Source: CAD feature listing. Evaluate the final solid. Frame: model axes, mm. Face numbers are marked on the shaded views. A direction names the side the tool comes from. Give positions to 0.01 mm unless a question says otherwise; leave off trailing zeros. Order: outer loops, then holes, each group sorted by start corner. A loop starts at its lowest first (then second) coordinate and runs counter-clockwise, first axis right, second up. Notation, with made-up numbers: M 67.5,31.5 L 89.5,31.5 A21 ccw 89.5,61.5 Z; hole C -24,70.25 d6. An arc over 180 degrees is marked long. Answer as a JSON object with one key per item and string values. Group by question number.
1. Material intervals for L1, parallel to Y at x = 4, z = 7; L2, parallel to X at y = 14.5, z = 15.5; L3, parallel to Y at x = -20, z = 5, sorted ascending. Write a range as [from, to].
2. Set-up query: the marked faces 1 and 2. Return all of +Z, -Z, +X, -X, +Y, -Y with unobstructed straight access to the full face (end or side cutting, diameter ignored); none if empty.
3. Section query B-B (x = -39.5). Output: boundary loops of the cut face in (y, z).
4. Section query A-A (z = 10.5). Output: boundary loops of the cut face in (x, y), plus the area to 3 significant figures.
5. Section query C-C (y = 182). Output: boundary loops of the cut face in (x, z).
6. Pin query (flat end, axial travel): P1, Ø2, axis at y = 113.5, z = 14, coming from the -X side; P2, Ø4, axis at x = -45, z = 13.5, coming from the +Y side; P3, Ø6, axis at x = -43, z = 25.5, coming from the +Y side; P4, Ø2.5, axis at x = 20, y = 19, coming from the -Z side. Return the tip coordinate at first contact, or that it passes through.
from build123d import *

# Parameters (mm, degrees)
SKETCH_1_R          = 1.5
EXTRUDE_1_DEPTH     = 30
SKETCH_2_R          = 1.5
CUT_EXTRUDE_1_DEPTH = 248.428255263
CUT_EXTRUDE_2_DEPTH = 248.428255263
SKETCH_4_R          = 1.5
CUT_EXTRUDE_3_DEPTH = 248.428255263


with BuildPart() as part:
    # 草图1 → 凸台-拉伸1 (new body)
    with BuildSketch(Plane.XY):
        with BuildLine():
            Line((2, 0), (22, 0))
            ThreePointArc((22, 0), (23.414213562, 0.585786438), (24, 2))
            Line((24, 2), (24, 220))
            Line((24, 220), (24, 233))
            ThreePointArc((24, 233), (23.414213562, 234.414213562), (22, 235))
            Line((22, 235), (0.195482884, 235))
            ThreePointArc((0.195482884, 235), (0.000927124, 234.990514521), (-0.19178318, 234.962148057))
            Line((-0.19178318, 234.962148057), (-70.981279128, 220.990537014))
            ThreePointArc((-70.981279128, 220.990537014), (-71.382091243, 220.45136106), (-70.884462612, 220))
            Line((-70.884462612, 220), (0, 220))
            Line((0, 220), (0, 2))
            ThreePointArc((0, 2), (0.585786438, 0.585786438), (2, 0))
        make_face()
        with Locations((20, 3)):
            Circle(SKETCH_1_R, mode=Mode.SUBTRACT)
        with Locations((4, 3)):
            Circle(SKETCH_1_R, mode=Mode.SUBTRACT)
        with Locations((4, 19)):
            Circle(SKETCH_1_R, mode=Mode.SUBTRACT)
    extrude(amount=EXTRUDE_1_DEPTH)

    # 草图2 → 切除-拉伸1 (cut, through all)
    with BuildSketch(Plane.XY.offset(30)):
        with Locations((20, 19)):
            Circle(SKETCH_2_R)
    extrude(amount=-CUT_EXTRUDE_1_DEPTH, mode=Mode.SUBTRACT)

    # 草图3 → 切除-拉伸2 (cut, through all)
    with BuildSketch(Plane(origin=(0, 0, 0), x_dir=(-1, 0, 0), z_dir=(0, 0, -1))):
        Polygon((-24, 30), (-11.097741442, 235), (-26.866932521, 235), align=None)
    extrude(amount=-CUT_EXTRUDE_2_DEPTH, mode=Mode.SUBTRACT)

    # 草图4 → 切除-拉伸3 (cut, through all)
    with BuildSketch(Plane(origin=(0, 0, 0), x_dir=(-1, 0, 0), z_dir=(0, 0, -1))):
        with Locations((-4, 79)):
            Circle(SKETCH_4_R)
    extrude(amount=-CUT_EXTRUDE_3_DEPTH, mode=Mode.SUBTRACT)


solid = part.part
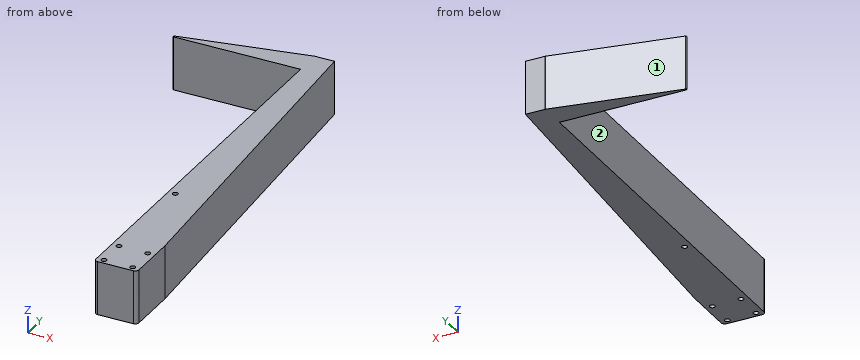
Answer sheet:
{
 "1": {"L1": "[0, 1.5], [4.5, 17.5], [20.5, 77.5], [80.5, 235]", "L2": "[0, 24]", "L3": "[220, 231.05]"},
 "2": {"face 1": "+Z, -Z, -X, +Y", "face 2": "+Z, -Z, -X, -Y"},
 "3": {"outline": "M 220,0 L 227.2,0 L 227.2,30 L 220,30 Z"},
 "4": {"outline": "M -70.98,220.99 A0.5 ccw -70.88,220 L 0,220 L 0,2 A2 ccw 2,0 L 22,0 A2 ccw 24,2 L 24,30 L 11.1,235 L 0.2,235 A2 ccw -0.19,234.96 Z; hole C 4,3 d3; hole C 4,19 d3; hole C 4,79 d3; hole C 20,3 d3; hole C 20,19 d3", "area": "4,850 mm^2"},
 "5": {"outline": "M 0,0 L 14.43,0 L 14.43,30 L 0,30 Z"},
 "6": {"P1": "x = 0", "P2": "y = 226.51", "P3": "y = 227.11", "P4": "through"}
}
